```python
from build123d import *

# Parameters (mm, degrees)
ESTRUSIONE_ESTRUSIONE1_DEPTH = 10
RACCORDO1_R                  = 3
FORO_FILETTATO_M3X0_5_1_D    = 2.5


with BuildPart() as part:
    # Schizzo1 → Estrusione-Estrusione1 (new body)
    with BuildSketch(Plane.XY):
        Polygon((-6, 0), (6, 0), (6, -3), (3, -3), (3, -6), (9, -6), (9, 3), (-6, 3), align=None)
    extrude(amount=ESTRUSIONE_ESTRUSIONE1_DEPTH)

    # Raccordo1
    raccordo1_edges = [part.edges().sort_by_distance(p)[0] for p in [
        (9, 3, 5),
        (9, -6, 5),
        (9, -1.5, 10),
        (9, -1.5, 0),
    ]]
    fillet(raccordo1_edges, radius=RACCORDO1_R - 0.0001)  # a hair under: the kernel refuses the full size

    # Foro filettato M3x0.5-1 (through all)
    with Locations(Plane(origin=(0, 3, 0), x_dir=(1, 0, 0), z_dir=(0, 1, 0))):
        with Locations((-3.5, -5)):
            Hole(FORO_FILETTATO_M3X0_5_1_D / 2)


solid = part.part
```
Work out the finished part from the listing and answer in its coordinate system (mm). A direction names the side the tool comes from. Give positions to 0.01 mm unless a question says otherwise; leave off trailing zeros. Write each loop counter-clockwise with the first axis right and the second up, starting at its lowest first coordinate (ties: lowest second). Pieces come first, ordered by that corner, then holes. Notation, with made-up numbers: (25.5, 65) -> (56.5, 65) arc R23 cw to (56.5, 77) -> close; hole circle Ø5 at (43.25, 73). An arc over 180 degrees is marked (long way). Write each question's results on one line, items separated by ' | '.
1. A tool of negligible diameter and unlimited length cuts with its end or side. For faces 1 (the flat face through (3, -4, 5)), 2 (the flat face through (5, -3, 5)), 3 (the cylindrical face through (7.69, -5.48, 5.07)), from which of +Z, -Z, +X, -X, +Y, -Y can it reach the whole face along a straight path? Write none if from no direction.
Data:
face 1: +Z, -Z, -X, -Y | face 2: +Z, -Z, -X | face 3: +Z, -Z, +X, -Y
2. Straight lines are drawn through the part: L1, parallel to Z at x = -3.5, y = 0.7; L2, parallel to Y at x = 3.75, z = 8; L3, parallel to Y at x = -5, z = 7.25. For each, find the intervals that lie inside material, in ascending order.
Data:
L1: 0 to 3.75, 6.25 to 10 | L2: -6 to -3, 0 to 3 | L3: 0 to 3
3. Determine the mould class of faces 4 (the flat face through (1, 1, 0)), 5 (the flat face through (4, -6, 5)), 6 (the flat face through (0, 0, 5)) for opening direction Y: +Y half, -Y half, draft (parallel to the pull), parting line (faces both ways), or undercut.
Data:
face 4: draft | face 5: -Y half | face 6: undercut
4. Find section C-C on x = 3.5. Determine the outline of the cut face in (y, z), and give its area (3 significant figures).
Data:
outline: (-6, 0) -> (-3, 0) -> (-3, 10) -> (-6, 10) -> close; (0, 0) -> (3, 0) -> (3, 10) -> (0, 10) -> close | area: 60.0 mm^2
5. Find section B-B on z = 5. Determine the outline of the cut face in (x, y).
Data:
outline: (-6, 0) -> (-4.75, 0) -> (-4.75, 3) -> (-6, 3) -> close; (-2.25, 0) -> (6, 0) -> (6, -3) -> (3, -3) -> (3, -6) -> (6, -6) arc R3 ccw to (9, -3) -> (9, 0) arc R3 ccw to (6, 3) -> (-2.25, 3) -> close
6. Find section A-A on x = -3.5. Determine the outline of the cut face in (y, z), and give its area (3 significant figures).
Data:
outline: (0, 0) -> (3, 0) -> (3, 3.75) -> (0, 3.75) -> close; (0, 6.25) -> (3, 6.25) -> (3, 10) -> (0, 10) -> close | area: 22.5 mm^2
7. Each of these flat-tipped pins is pushed along its axis until it touches: pin 1 Ø1 at (y, z) = (0.5, 1.5) entering from +X; pin 2 Ø3 at (x, z) = (-3, 9) entering from -Y; pin 3 Ø0.9 at (y, z) = (-1, 3) entering from -X. Where does it stop, or does it pass through?
Data:
pin 1: x = 8.83 | pin 2: y = 0 | pin 3: x = 6
8. Find section D-D on y = 2. Determine the outline of the cut face in (x, z).
Data:
outline: (-6, 0) -> (6, 0) arc R3 ccw to (8.24, 1) -> (8.24, 9) arc R3 ccw to (6, 10) -> (-6, 10) -> close; hole circle Ø2.5 at (-3.5, 5)
